```python
from build123d import *

# Parameters (mm, degrees)
SKETCH1_RX           = 800
SKETCH1_RY           = 250
SKETCH1_R            = 62.5
BOSS_EXTRUDE1_DEPTH  = 150
BOSS_EXTRUDE9_DEPTH  = 150
SKETCH17_R           = 225
BOSS_EXTRUDE13_DEPTH = 450


with BuildPart() as part:
    # Sketch1 → Boss-Extrude1 (new body)
    with BuildSketch(Plane.XY):
        with Locations((-931.832148188, 736.166079396)):
            Ellipse(SKETCH1_RX, SKETCH1_RY)
        with Locations((-1619.332148188, 736.166079396)):
            Circle(SKETCH1_R, mode=Mode.SUBTRACT)
        with Locations((-244.332148188, 736.166079396)):
            Circle(SKETCH1_R, mode=Mode.SUBTRACT)
    extrude(amount=BOSS_EXTRUDE1_DEPTH)

    # Sketch12 → Boss-Extrude9 (add)
    with BuildSketch(Plane(origin=(0, 0, 0), x_dir=(-1, 0, 0), z_dir=(0, 0, -1))):
        Polygon((991.0872246, 633.924307933), (1050.003657809, 736.361595141), (990.748581397, 838.603366603), (872.577071776, 838.407850859), (813.660638567, 735.970563652), (872.915714979, 633.728792189), align=None)
    extrude(amount=BOSS_EXTRUDE9_DEPTH)

    # Sketch17 → Boss-Extrude13 (add)
    with BuildSketch(Plane(origin=(0, 0, 0), x_dir=(-1, 0, 0), z_dir=(0, 0, -1))):
        with Locations(Location((931.832148188, 736.166079396, 0), (0, 0, 180))):
            Circle(SKETCH17_R)
        Polygon((991.0872246, 633.924307933), (1050.003657809, 736.361595141), (990.748581397, 838.603366603), (872.577071776, 838.407850859), (813.660638567, 735.970563652), (872.915714979, 633.728792189), align=None, mode=Mode.SUBTRACT)
    extrude(amount=BOSS_EXTRUDE13_DEPTH)


solid = part.part
```
Geometry check sheet. Reference: the model listing, model coordinates, mm. A direction names the side the tool comes from. Round coordinates to 2 decimals unless told otherwise and drop trailing zeros. Loops run counter-clockwise (first coordinate to the right, second up) from the corner with the lowest first, then second, coordinate; pieces in that order, holes last. Notation, with made-up numbers: M 8.5,-34.75 L 66.5,-34.75 A26 cw 66.5,-9.75 Z; hole C -35,55 d4. An arc over 180 degrees is marked long. Return JSON: item names as keys, results as strings. Group by question number.
(1) Mould release check, pull along X, two halves, no side actions. Record for faces 1 (the face through (-252.468, 798.134, 73.95)), 2 (the face through (-943, 962, 0)), 3 (the face through (-1156.615, 726.273, -221.85)): pulls with the +X half, pulls with the -X half, needs draft (parallel to the pull), parting line crosses it, or undercut.
(2) Go/stop test with flat-tipped pins: pin 1 (1 mm diameter, centred on x = -776.5, z = -82.5, fed in from -Y); pin 2 (6 mm diameter, centred on y = 836, z = -68, fed in from -X); pin 3 (2 mm diameter, centred on x = -537.5, y = 712.5, fed in from -Z). Record where each tip stops, or that it passes through.
(3) Section check B-B, the plane z = -59. Enter the section's corners in (x, y), and give its area (3 significant figures).
(4) Scan lines: line 1 along X through (y, z) = (763, 2.5); line 2 along X through (y, z) = (771.5, -279.5); line 3 along X through (y, z) = (666.5, -385.5). Record each from-to range of solid material in increasing order. Write a range as [from, to].
(5) Section check C-C, the plane z = 61. Give the number of separate pieces and of enclosed holes in the cut face, and give its area (3 significant figures).
(6) Section check A-A, the plane z = -317. Enter the section's corners in (x, y), and give its area (3 significant figures).
(7) Set-up check for faces 4 (the face through (-1585.733, 788.866, 73.95)), 5 (the face through (-930, 738, -150)): record each of +Z, -Z, +X, -X, +Y, -Y from which the full face is reachable in a straight line by a thin tool's end or side.
Data:
{
 "1": {"face 1": "undercut", "face 2": "needs draft", "face 3": "parting line crosses it"},
 "2": {"pin 1": "y = 572.91", "pin 2": "x = -1134.93", "pin 3": "z = 0"},
 "3": {"outline": "C -931.83,736.17 d450", "area": "159,000 mm²"},
 "4": {"line 1": "[-1727.21, -1675.78], [-1562.89, -300.78], [-187.89, -136.45]", "line 2": "[-1154.04, -1029.64], [-834.1, -709.62]", "line 3": "[-1145.78, -1009.82], [-853.92, -717.89]"},
 "5": {"separate pieces": "1", "enclosed holes": "2", "area": "604,000 mm²"},
 "6": {"outline": "C -931.83,736.17 d450; hole M -1050,736.36 L -991.09,633.92 L -872.92,633.73 L -813.66,735.97 L -872.58,838.41 L -990.75,838.6 Z", "area": "123,000 mm²"},
 "7": {"face 4": "+Z, -Z", "face 5": "-Z"}
}
